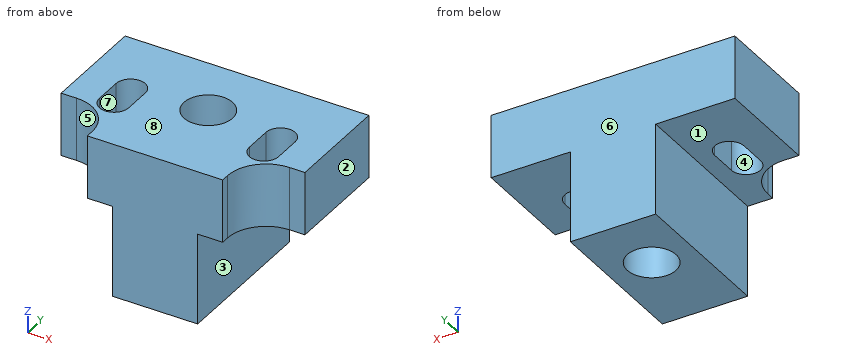
from build123d import *
from build123d.topology import SkipClean

# Parameters (mm, degrees)
BOSS_EXTRUDE1_DEPTH = 25
CUT_EXTRUDE1_DEPTH  = 41.867591072
SKETCH8_R           = 4
CUT_EXTRUDE2_DEPTH  = 41.867591072
CUT_EXTRUDE3_DEPTH  = 36.355339059


with BuildPart() as part:
    # Sketch6 → Boss-Extrude1 (new body)
    with BuildSketch(Plane(origin=(0, 0, 0), x_dir=(1, 0, 0), z_dir=(0, 1, 0))):
        Polygon((0, 0), (-20, 0), (-20, 10.4), (-7, 10.4), (-7, 25.4), (0, 25.4), align=None)
    extrude(amount=BOSS_EXTRUDE1_DEPTH)

    # Sketch7 → Cut-Extrude1 (cut, through all)
    with BuildSketch(Plane.XY):
        with BuildLine():
            Line((-9.9, 13.75), (-9.9, 9.25))
            ThreePointArc((-9.9, 9.25), (-12.3, 6.85), (-14.7, 9.25))
            Line((-14.7, 9.25), (-14.7, 13.75))
            ThreePointArc((-14.7, 13.75), (-12.3, 16.15), (-9.9, 13.75))
        make_face()
    extrude(amount=-CUT_EXTRUDE1_DEPTH, mode=Mode.SUBTRACT)

    # Sketch8 → Cut-Extrude2 (cut, through all)
    with BuildSketch(Plane.XY):
        with Locations((0, 14.49399695)):
            Circle(SKETCH8_R)
    extrude(amount=-CUT_EXTRUDE2_DEPTH, mode=Mode.SUBTRACT)

    # Sketch9 → Cut-Extrude3 (cut, through all)
    with BuildSketch(Plane(origin=(0, 0, -10.4), x_dir=(-1, 0, 0), z_dir=(0, 0, -1))):
        with BuildLine():
            Line((11.11, 0), (11.11, 1.27))
            ThreePointArc((11.11, 1.27), (12.969871939, 5.760128061), (17.46, 7.62))
            Line((17.46, 7.62), (20, 7.62))
            Line((20, 7.62), (20, 0))
            Line((20, 0), (11.11, 0))
        make_face()
    extrude(amount=-CUT_EXTRUDE3_DEPTH, mode=Mode.SUBTRACT)

    # Mirror1: part across plane


with BuildPart() as part_1:
    with SkipClean():  # the faces are left unmerged after this step: merging them gives an invalid solid
        add(part.part)
        add(part.part.mirror(Plane(origin=(0, 0, 0), x_dir=(0, 0, 1), z_dir=(1, 0, 0))))


solid = part_1.part
Verification items for the finished model (mm, model axes). Face numbers are marked on the shaded views. A direction names the side the tool comes from. Give positions to 0.01 mm unless a question says otherwise; leave off trailing zeros. Loops run counter-clockwise (first coordinate to the right, second up) from the corner with the lowest first, then second, coordinate; pieces in that order, holes last.
1. Release check for a two-part mould opening along Y. For the marked faces 5, 6, 7 and 8 record: +Y half, -Y half, draft (parallel to the pull), parting line (faces both ways), or undercut.
Derived:
face 5: -Y half
face 6: +Y half
face 7: undercut
face 8: draft
2. Cross-section at D-D on y = 21.5. Record the cut outline in (x, z), and give its area (3 significant figures).
Derived:
outline: (-20, -10.4) - (-7, -10.4) - (-7, -25.4) - (7, -25.4) - (7, -10.4) - (20, -10.4) - (20, 0) - (-20, 0) - close
area: 626 mm2
3. Material ranges on probe 1 along X at (y, z) = (14.25, -1); probe 2 along X at (y, z) = (13.25, -6); probe 3 along X at (y, z) = (18.75, -13.5), recorded low to high.
Derived:
probe 1: x = -20 to -14.65, -9.95 to -3.99, 3.99 to 9.95, 14.65 to 20
probe 2: x = -20 to -14.7, -9.9 to -3.8, 3.8 to 9.9, 14.7 to 20
probe 3: x = -7 to 7
4. Cross-section at B-B on x = -12.3. Record the cut outline in (y, z), and give its area (3 significant figures).
Derived:
outline: (4.97, -10.4) - (6.85, -10.4) - (6.85, 0) - (4.97, 0) - close; (16.15, -10.4) - (25, -10.4) - (25, 0) - (16.15, 0) - close
area: 112 mm2
5. Cross-section at C-C on z = -16.25. Record the cut outline in (x, y).
Derived:
outline: (-7, 0) - (7, 0) - (7, 25) - (-7, 25) - close; hole circle Ø8 at (0, 14.49)
6. Cross-section at A-A on z = -4.5. Record the cut outline in (x, y).
Derived:
outline: (-20, 7.62) - (-17.46, 7.62) arc R6.35 cw to (-11.11, 1.27) - (-11.11, 0) - (11.11, 0) - (11.11, 1.27) arc R6.35 cw to (17.46, 7.62) - (20, 7.62) - (20, 25) - (-20, 25) - close; hole (-14.7, 9.25) arc R2.4 ccw to (-9.9, 9.25) - (-9.9, 13.75) arc R2.4 ccw to (-14.7, 13.75) - close; hole circle Ø8 at (0, 14.49); hole (9.9, 9.25) arc R2.4 ccw to (14.7, 9.25) - (14.7, 13.75) arc R2.4 ccw to (9.9, 13.75) - close
7. Go/stop test with flat-tipped pins: P1, Ø5, axis at x = 0, y = 14.49, coming from the +Z side; P2, Ø7.5, axis at y = 6.5, z = -20, coming from the +X side; P3, Ø4, axis at x = -11.5, y = 6.5, coming from the -Z side; P4, Ø1, axis at y = 1, z = -2.5, coming from the +X side. Record where each tip stops, or that it passes through.
Derived:
P1: passes through
P2: stops at x = 7
P3: stops at z = -10.4
P4: stops at x = 11.11
8. Tool access check on the marked faces 1, 2, 3 and 4. Record the directions out of +Z, -Z, +X, -X, +Y, -Y that give a thin tool (end or side, any length) a straight path to the whole face; none if there is none.
Derived:
face 1: -Z, -X, +Y, -Y
face 2: +Z, -Z, +X, +Y, -Y
face 3: -Z, +X, +Y, -Y
face 4: +Z, -Z
